Design review of the part built by this model. Coordinates are the model's own, in mm. Face numbers are marked on the shaded views. A direction names the side the tool comes from. Coordinates: 2 decimals unless noted, no trailing zeros. Loops run counter-clockwise (first coordinate to the right, second up) from the corner with the lowest first, then second, coordinate; pieces in that order, holes last. Notation, with made-up numbers: (-9, -3) -> (31, -3) arc R22 cw to (31, 12) -> close; hole circle Ø3 at (-20, 37). An arc over 180 degrees is marked (long way). Use one line per item in the form item = value. Start each with the question number.
1. Consider section D-D (x = 64). State the section outline as (y, z) points, then the cut area to 3 significant figures.
2. The part is to be moulded in two halves that separate along X. For the marked faces 3, 4, 5 and 6, say which applies: released by +X, released by -X, zero draft, split by the parting line, or undercut.
3. Consider section B-B (y = 29.5). State the section outline as (x, z) points, then the cut area to 3 significant figures.
4. Wall thickness on line 1 (X direction, y = 21.5, z = -19.5); line 2 (Y direction, x = 1, z = -4); line 3 (Z direction, x = 13, y = 50.5): over which ranges is each line inside the solid? List them lowest first. Write a range as from..to.
5. Consider section A-A (z = -7). State the section outline as (x, y) points, then the cut area to 3 significant figures.
6. For pin 1 (0.8 mm diameter, centred on y = 1, z = 1, fed in from -X); pin 2 (2.5 mm diameter, centred on x = 35, z = 1, fed in from +Y); pin 3 (2.5 mm diameter, centred on x = 83.38, y = 55.19, fed in from -Z), all flat-tipped, find the tip position at first contact; note any pin that passes through.
7. Consider section C-C (x = 11.5). State the section outline as (y, z) points, then the cut area to 3 significant figures.
8. Machinability: for the marked faces 1 and 2, which of the approach directions +Z, -Z, +X, -X, +Y, -Y give a long, thin tool a straight path to every point of the face, cutting with its end or side? Answer none if there is none.
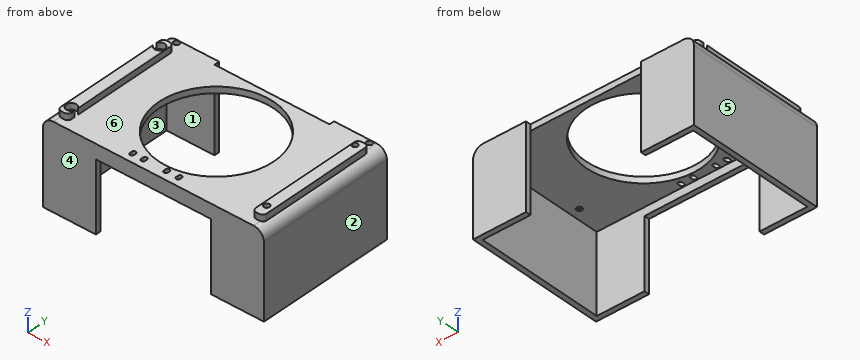
Autodesk Inventor part; units mm, degrees
ref_plane "YZ Plane" through (0, 0, 0) normal (1, 0, 0) x (0, 1, 0)
ref_plane "XZ Plane" through (0, 0, 0) normal (0, 1, 0) x (-1, 0, 0)
ref_plane "XY Plane" through (0, 0, 0) normal (0, 0, 1) x (1, 0, 0)
sketch "Sketch1" plane through (0, 0, 0) normal (0, 0, 1) x (1, 0, 0)
  circle A0 centre (37.2069, 31.0185) radius 28
  line L0 (-13.5931, 3.1035) -> (88.0069, 3.1035) construction
  line L1 (14.2069, 60.2535) -> (-13.5931, 60.2535) construction
  line L2 (88.0069, 60.2535) -> (60.0869, 60.2535) construction
  line L3 (88.0069, 3.1035) -> (88.0069, 60.2535) construction
  line L4 (-13.5931, 60.2535) -> (-13.5931, 3.1035) construction
  line L5 (11.269, 60.2207) -> (67.149, 60.2207) construction
  line L6 (67.149, 60.2207) -> (67.149, 72.2207) construction
  line L7 (67.149, 72.2207) -> (11.269, 72.2207) construction
  line L8 (11.269, 72.2207) -> (11.269, 60.2207) construction
  circle A1 centre (61.389, 6.2635) radius 1.5 construction
  circle A2 centre (61.389, 55.7935) radius 1.5 construction
  circle A3 centre (5.509, 55.7935) radius 1.5 construction
  circle A4 centre (11.269, 6.9135) radius 1.5 construction
  arc A5 (11.269, 7.6907) -> (11.269, 1.6907) centre (11.269, 4.6907) ccw construction
  line L9 (11.269, 1.6907) -> (11.269, -3.7465) construction
  line L10 (11.269, -3.7465) -> (67.149, -3.7465) construction
  line L11 (67.149, -3.7465) -> (67.149, 1.6907) construction
  arc A6 (67.149, 1.6907) -> (67.149, 7.6907) centre (67.149, 4.6907) ccw construction
  line L12 (67.149, 7.6907) -> (67.149, 51.2207) construction
  arc A7 (67.149, 51.2207) -> (67.149, 57.2207) centre (67.149, 54.2207) ccw construction
  line L13 (67.149, 57.2207) -> (67.149, 60.2207) construction
  line L14 (67.149, 60.2207) -> (11.269, 60.2207) construction
  line L15 (11.269, 60.2207) -> (11.269, 57.2207) construction
  arc A8 (11.269, 57.2207) -> (11.269, 51.2207) centre (11.269, 54.2207) ccw construction
  line L16 (11.269, 51.2207) -> (11.269, 7.6907) construction
  line L17 (-16.5931, -3.7465) -> (91.0069, -3.7465)
  line L18 (91.0069, -3.7465) -> (91.0069, 64.2535)
  line L19 (91.0069, 64.2535) -> (-16.5931, 64.2535)
  line L20 (-16.5931, 64.2535) -> (-16.5931, -3.7465)
  line L21 (37.2069, -3.7465) -> (37.2069, 64.2535) construction
  circle A9 centre (37.2069, 31.0185) radius 23
  point P0 (0, 0)
  dimension "d42" = 0
  dimension "d43" = 3
  dimension "d44" = 3
  dimension "d45" = 4
  dimension "d46" = 4
  dimension "d47" = 57.15
  dimension "d48" = 57.15
  dimension "d49" = 101.6
  dimension "d50" = 3.81
  dimension "d56" = 68
  dimension "d59" = 56
extrude "Extrusion1" add sketch "Sketch1" along normal blind 3 contours L20 L19 L18 L17
sketch "Sketch2" plane through (0, 0, 0) normal (0, 0, -1) x (-1, 0, 0)
  circle A0 centre (-37.2069, 31.0185) radius 28
  line L0 (16.5931, -3.7465) -> (-91.0069, -3.7465)
  line L1 (16.5931, 64.2535) -> (16.5931, -3.7465)
  line L2 (-91.0069, 64.2535) -> (16.5931, 64.2535)
  line L3 (-91.0069, -3.7465) -> (-91.0069, 64.2535)
  line L4 (-88.5069, 61.7535) -> (14.0931, 61.7535)
  line L5 (14.0931, 61.7535) -> (14.0931, -1.2465)
  line L6 (14.0931, -1.2465) -> (-88.5069, -1.2465)
  line L7 (-88.5069, -1.2465) -> (-88.5069, 61.7535)
  dimension "d51" = 2.5
  dimension "d52" = 2.5
  dimension "d53" = 2.5
  dimension "d54" = 2.5
extrude "Extrusion2" add sketch "Sketch2" along normal blind 38 contours L0 L3 L2 L1
sketch "Sketch4" plane through (0, 0, 3) normal (0, 0, 1) x (1, 0, 0)
  ellipse E0 centre (83.8034, 62.7427) end of major axis (82.4034, 62.7427) minor radius 1.3886
  ellipse E1 centre (83.8006, 13.6146) end of major axis (82.4006, 13.6146) minor radius 1.3886
  ellipse E2 centre (-10.1794, 13.6199) end of major axis (-11.5794, 13.6199) minor radius 1.3886
  ellipse E3 centre (-10.1766, 62.7479) end of major axis (-11.5766, 62.7479) minor radius 1.3886
  point P0 (0, 0)
extrude "Extrusion3" cut sketch "Sketch4" against normal blind 3
chamfer "Chamfer1" [suppressed]
sketch "Sketch5" plane through (-16.5931, 64.2535, 3) normal (0, 1, 0) x (1, 0, 0)
  line L0 (0, 0) -> (107.6, 0)
  line L1 (25.8, 63) -> (81.8, 63)
  line L2 (81.8, 63) -> (81.8, 7)
  line L3 (81.8, 7) -> (25.8, 7)
  line L4 (25.8, 7) -> (25.8, 63)
  line L5 (53.8, 0) -> (53.8, -31.7336) construction
  line L6 (25.8, 63) -> (81.8, 7) construction
  line L7 (81.8, 63) -> (25.8, 7) construction
  line L8 (104.9242, 0) -> (-0.6758, 0)
  line L9 (107.6, 0) -> (0, 0)
  line L10 (0, 41) -> (107.6, 41)
  line L11 (53.8, 41) -> (53.8, 0) construction
  point P0 (19.351, -30)
  point P1 (53.8, 35)
  point P2 (53.8, 35)
  dimension "d28" = 56
  dimension "d29" = 56
  dimension "d41" = 7
extrude "Extrusion4" cut sketch "Sketch5" against normal blind 100
fillet "Fillet2" radius 5 2 edges at (-16.5931, 30.2535, 3) (91.0069, 30.2535, 3)
fillet "Fillet3" [suppressed]
sketch "Sketch6" plane through (9.2069, 64.2535, -4) normal (0, 1, 0) x (1, 0, 0)
  line L0 (81.8, -7) -> (-25.8, -7)
  line L1 (0, 0) -> (56, 0)
  line L2 (56, 0) -> (56, -7)
  line L3 (56, -7) -> (0, -7)
  line L4 (0, -7) -> (0, 0)
  point P0 (76.8, -7)
  point P1 (-20.8, -7)
  point P2 (-9.2069, -4)
extrude "Extrusion5" cut sketch "Sketch6" against normal blind 2.5
sketch "Sketch7" plane through (0, 0, 3) normal (0, 0, 1) x (1, 0, 0)
  line L0 (-16.5931, -3.7465) -> (91.0069, -3.7465)
  line L1 (65.2069, 61.7535) -> (9.2069, 61.7535)
  line L2 (37.2069, -3.7465) -> (37.2069, 61.7535) construction
  line L3 (23.1969, -0.7465) -> (23.1969, -0.7465)
  line L4 (22.1969, 0.2535) -> (22.1969, 1.2535)
  line L5 (23.1969, 2.2535) -> (23.1969, 2.2535)
  line L6 (24.1969, 1.2535) -> (24.1969, 0.2535)
  arc A0 (24.1969, 1.2535) -> (23.1969, 2.2535) centre (23.1969, 1.2535) ccw
  arc A1 (23.1969, 2.2535) -> (22.1969, 1.2535) centre (23.1969, 1.2535) ccw
  arc A2 (22.1969, 0.2535) -> (23.1969, -0.7465) centre (23.1969, 0.2535) ccw
  arc A3 (23.1969, -0.7465) -> (24.1969, 0.2535) centre (23.1969, 0.2535) ccw
  line L7 (27.6969, 0.2535) -> (27.6969, 1.2535)
  line L8 (29.6969, 1.2535) -> (29.6969, 0.2535)
  arc A4 (29.6969, 1.2535) -> (28.6969, 2.2535) centre (28.6969, 1.2535) ccw
  arc A5 (28.6969, 2.2535) -> (27.6969, 1.2535) centre (28.6969, 1.2535) ccw
  arc A6 (27.6969, 0.2535) -> (28.6969, -0.7465) centre (28.6969, 0.2535) ccw
  arc A7 (28.6969, -0.7465) -> (29.6969, 0.2535) centre (28.6969, 0.2535) ccw
  line L9 (44.7169, 0.2535) -> (44.7169, 1.2535)
  line L10 (46.7169, 1.2535) -> (46.7169, 0.2535)
  arc A8 (46.7169, 1.2535) -> (45.7169, 2.2535) centre (45.7169, 1.2535) ccw
  arc A9 (45.7169, 2.2535) -> (44.7169, 1.2535) centre (45.7169, 1.2535) ccw
  arc A10 (44.7169, 0.2535) -> (45.7169, -0.7465) centre (45.7169, 0.2535) ccw
  arc A11 (45.7169, -0.7465) -> (46.7169, 0.2535) centre (45.7169, 0.2535) ccw
  line L11 (38.6969, 0.2535) -> (38.6969, 1.2535)
  line L12 (40.6969, 1.2535) -> (40.6969, 0.2535)
  arc A12 (40.6969, 1.2535) -> (39.6969, 2.2535) centre (39.6969, 1.2535) ccw
  arc A13 (39.6969, 2.2535) -> (38.6969, 1.2535) centre (39.6969, 1.2535) ccw
  arc A14 (38.6969, 0.2535) -> (39.6969, -0.7465) centre (39.6969, 0.2535) ccw
  arc A15 (39.6969, -0.7465) -> (40.6969, 0.2535) centre (39.6969, 0.2535) ccw
  line L13 (29.6969, 0.7535) -> (44.7169, 0.7535) construction
  point P0 (-11.5931, -3.7465)
  point P1 (86.0069, -3.7465)
  point P2 (0, 0)
  point P3 (24.1969, -0.7465)
  point P4 (22.1969, 2.2535)
  point P5 (24.1969, 2.2535)
  point P6 (29.6969, -0.7465)
  point P7 (27.6969, 2.2535)
  point P8 (29.6969, 2.2535)
  point P9 (46.7169, -0.7465)
  point P10 (44.7169, 2.2535)
  point P11 (46.7169, 2.2535)
  point P12 (40.6969, -0.7465)
  point P13 (38.6969, 2.2535)
  point P14 (40.6969, 2.2535)
  point P15 (37.2069, 0.7535)
  dimension "d64" = 2
  dimension "d66" = 3
  dimension "d67" = 1
  dimension "d68" = 1
  dimension "d69" = 4
  dimension "d78" = 16.5
  dimension "d79" = 13.01
  dimension "d80" = 1.49
extrude "Extrusion6" cut sketch "Sketch7" against normal blind 3
sketch "Sketch10" plane through (0, 0, 3) normal (0, 0, 1) x (1, 0, 0)
  circle A0 centre (37.2069, 31.0185) radius 28
  circle A1 centre (83.3776, 55.1949) radius 1.4
  circle A2 centre (-9.9042, 4.3621) radius 1.4
  circle A3 centre (-10.5933, 53.8873) radius 1.4
  circle A4 centre (84.0667, 5.6697) radius 1.4
  line L0 (-9.5933, 58.2873) -> (-10.9042, 58.2873)
  line L1 (-12.9042, 56.2873) -> (-12.9042, 1.9621)
  line L2 (-10.9042, -0.0379) -> (-9.5933, -0.0379)
  line L3 (-7.5933, 1.9621) -> (-7.5933, 56.2873)
  arc A5 (-7.5933, 56.2873) -> (-9.5933, 58.2873) centre (-9.5933, 56.2873) ccw
  arc A6 (-10.9042, 58.2873) -> (-12.9042, 56.2873) centre (-10.9042, 56.2873) ccw
  arc A7 (-9.5933, -0.0379) -> (-7.5933, 1.9621) centre (-9.5933, 1.9621) ccw
  arc A8 (-12.9042, 1.9621) -> (-10.9042, -0.0379) centre (-10.9042, 1.9621) ccw
  line L4 (37.2069, 31.0185) -> (37.2069, 47.569) construction
  line L5 (84.0072, 58.2873) -> (85.3181, 58.2873)
  line L6 (87.3181, 56.2873) -> (87.3181, 1.9621)
  line L7 (85.3181, -0.0379) -> (84.0072, -0.0379)
  line L8 (82.0072, 1.9621) -> (82.0072, 56.2873)
  arc A9 (84.0072, 58.2873) -> (82.0072, 56.2873) centre (84.0072, 56.2873) ccw
  arc A10 (87.3181, 56.2873) -> (85.3181, 58.2873) centre (85.3181, 56.2873) ccw
  arc A11 (82.0072, 1.9621) -> (84.0072, -0.0379) centre (84.0072, 1.9621) ccw
  arc A12 (85.3181, -0.0379) -> (87.3181, 1.9621) centre (85.3181, 1.9621) ccw
  point P0 (0, 0)
  dimension "d101" = 3
  dimension "d103" = 3
  dimension "d104" = 3
  dimension "d105" = 3
  dimension "d106" = 2
  dimension "d107" = 2
extrude "Extrusion9" add sketch "Sketch10" along normal blind 3 and the other way blind 2 contours A1 L8 A9 L5 A10 L6 A12 L7 A11 | A5 L3 A7 L2 A8 L1 A6 L0
sketch "Sketch11" plane through (0, 0, 6) normal (0, 0, 1) x (1, 0, 0)
  circle A0 centre (-10.5933, 53.8873) radius 1.4
  circle A1 centre (-9.9042, 4.3621) radius 1.4
  line L0 (82.0072, 54.9087) -> (82.0072, 1.9621)
  arc A2 (82.0072, 1.9621) -> (84.0072, -0.0379) centre (84.0072, 1.9621) ccw
  line L1 (84.0072, -0.0379) -> (85.3181, -0.0379)
  arc A3 (85.3181, -0.0379) -> (87.3181, 1.9621) centre (85.3181, 1.9621) ccw
  line L2 (87.3181, 1.9621) -> (87.3181, 56.2873)
  arc A4 (87.3181, 56.2873) -> (85.3181, 58.2873) centre (85.3181, 56.2873) ccw
  line L3 (85.3181, 58.2873) -> (84.0072, 58.2873)
  arc A5 (84.0072, 58.2873) -> (82.0072, 56.2873) centre (84.0072, 56.2873) ccw
  circle A6 centre (-10.5933, 53.8873) radius 2.5
  circle A7 centre (-9.9042, 4.3621) radius 2.5
  circle A8 centre (78.5569, 55.7835) radius 2.5
  circle A9 centre (78.5569, 6.2535) radius 2.5
  arc A10 (82.0072, 54.9087) -> (82.0072, 55.4811) centre (83.3776, 55.1949) ccw
  line L4 (82.0072, 56.2873) -> (82.0072, 55.4811)
  point P0 (0, 0)
  dimension "d112" = 5
  dimension "d114" = 5
  dimension "d115" = 5
  dimension "d116" = 5
extrude "Extrusion10" cut sketch "Sketch11" against normal blind 3 contours A0 | A1 | A6 | A7 | A8 | A9
properties part number "Enclosure01"
Geometry check:
q1.outline = (-3.75, -4) -> (-1.25, -4) -> (-1.25, 0) -> (22.89, 0) -> (22.89, 3) -> (-3.75, 3) -> close; (39.15, 0) -> (61.75, 0) -> (61.75, 3) -> (39.15, 3) -> close
q1.area = 158 mm²
q2.face_3 = undercut
q2.face_4 = zero draft
q2.face_5 = released by -X
q2.face_6 = undercut
q3.outline = (-16.59, -38) -> (-14.09, -38) -> (-14.09, 0) -> (9.25, 0) -> (9.25, 3) -> (-7.59, 3) -> (-7.59, 6) -> (-12.9, 6) -> (-12.9, 2.83) arc R5 ccw to (-16.59, -2) -> close; (65.17, 0) -> (88.51, 0) -> (88.51, -38) -> (91.01, -38) -> (91.01, -2) arc R5 ccw to (87.32, 2.83) -> (87.32, 6) -> (82.01, 6) -> (82.01, 3) -> (65.17, 3) -> close
q3.area = 366 mm²
q4.line_1 = -16.59..-14.09, 88.51..91.01
q4.line_2 = -3.75..-1.25, 61.75..64.25
q4.line_3 = 0..3
q5.outline = (-16.59, -3.75) -> (9.21, -3.75) -> (9.21, -1.25) -> (-14.09, -1.25) -> (-14.09, 61.75) -> (9.21, 61.75) -> (9.21, 64.25) -> (-16.59, 64.25) -> close; (65.21, -3.75) -> (91.01, -3.75) -> (91.01, 64.25) -> (65.21, 64.25) -> (65.21, 61.75) -> (88.51, 61.75) -> (88.51, -1.25) -> (65.21, -1.25) -> close
q5.area = 573 mm²
q6.pin_1 = -15.86
q6.pin_2 = 61.75
q6.pin_3 = 0
q7.outline = (-3.75, -4) -> (-1.25, -4) -> (-1.25, 0) -> (19.92, 0) -> (19.92, 3) -> (-3.75, 3) -> close; (42.12, 0) -> (61.75, 0) -> (61.75, 3) -> (42.12, 3) -> close
q7.area = 140 mm²
q8.face_1 = -Z
q8.face_2 = +Z, -Z, +X, +Y, -Y
